Autodesk Inventor part; units mm, degrees
ref_plane "YZ Plane" through (0, 0, 0) normal (1, 0, 0) x (0, 1, 0)
ref_plane "XZ Plane" through (0, 0, 0) normal (0, 1, 0) x (-1, 0, 0)
ref_plane "XY Plane" through (0, 0, 0) normal (0, 0, 1) x (1, 0, 0)
sketch "Esboço1" plane through (0, 0, 0) normal (0, 1, 0) x (-1, 0, 0)
  line L0 (0, 0) -> (0, -150)
  line L1 (0, -150) -> (100, -150)
  line L2 (100, -150) -> (100, 0)
  line L3 (100, 0) -> (0, 0)
  dimension "d0" = 150
  dimension "d1" = 100
extrude "Extrusão1" add sketch "Esboço1" along normal blind 5
fillet "Arredondamento1" radius 5 1 edges at (0, 2.5, 0)
fillet "Arredondamento2" radius 5 1 edges at (-100, 2.5, 0)
fillet "Arredondamento3" radius 5 2 edges at (-100, 2.5, -150) (0, 2.5, -150)
sketch "Esboço2" plane through (0, 5, 0) normal (0, 1, 0) x (1, 0, 0)
  circle A0 centre (-5, 5) radius 2.5
  circle A1 centre (-95, 5) radius 2.5
  circle A2 centre (-68, 145) radius 2.5
  circle A3 centre (-32, 145) radius 2.5
  circle A4 centre (-5, 5) radius 2.5
  dimension "d26" = 5
  dimension "d28" = 5
  dimension "d41" = 5
  dimension "d42" = 5
sketch "Esboço3" plane through (0, 5, 0) normal (0, 1, 0) x (1, 0, 0)
  line L0 (-5, 150) -> (-95, 150)
  line L1 (-80, 108) -> (-80, 63)
  line L2 (-100, 145) -> (-100, 5)
  line L3 (-80, 108) -> (-106.6116, 108)
  line L4 (-80, 63) -> (-106.6116, 63)
  circle A0 centre (-32, 145) radius 2.5
  line L5 (-67.9453, 145) -> (-32, 145)
  point P0 (0, 0)
  point P1 (-100, 108)
  point P2 (-100, 63)
  point P3 (-100, 108)
  point P4 (-100, 63)
  dimension "d53" = 45
extrude "Extrusão9" cut sketch "Esboço3" against normal through all contours L1 L4 L2 L3
extrude "Extrusão10" cut sketch "Esboço2" against normal through all
sketch "Esboço4" plane through (0, 5, 0) normal (0, 1, 0) x (1, 0, 0)
  line L0 (-95, 0) -> (-5, 0)
  line L1 (-5, 34.9997) -> (-42.3, 34.9997)
  line L2 (-42.3, 12.0997) -> (-5, 12.0997)
  line L3 (-42.3, 12.0997) -> (-42.3, 9.7997)
  line L4 (-42.3, 9.7997) -> (-5, 9.7997)
  line L5 (-5, 9.7997) -> (-5, 12.0997)
  line L6 (-5, 34.9997) -> (-5, 37.2997)
  line L7 (-5, 37.2997) -> (-42.3, 37.2997)
  line L8 (-42.3, 37.2997) -> (-42.3, 34.9997)
  line L9 (-57.3, 34.9997) -> (-94.6, 34.9997)
  line L10 (-94.6, 12.0997) -> (-57.3, 12.0997)
  line L11 (-94.6, 12.0997) -> (-94.6, 9.7997)
  line L12 (-94.6, 9.7997) -> (-57.3, 9.7997)
  line L13 (-57.3, 9.7997) -> (-57.3, 12.0997)
  line L14 (-57.3, 34.9997) -> (-57.3, 37.2997)
  line L15 (-57.3, 37.2997) -> (-94.6, 37.2997)
  line L16 (-94.6, 37.2997) -> (-94.6, 34.9997)
  point P0 (0, 0)
  dimension "d62" = 37.3
  dimension "d63" = 22.9
  dimension "d64" = 2.3
  dimension "d65" = 2.3
  dimension "d67" = 37.3
extrude "Extrusão11" cut sketch "Esboço4" against normal through all
properties part number "BaseS"
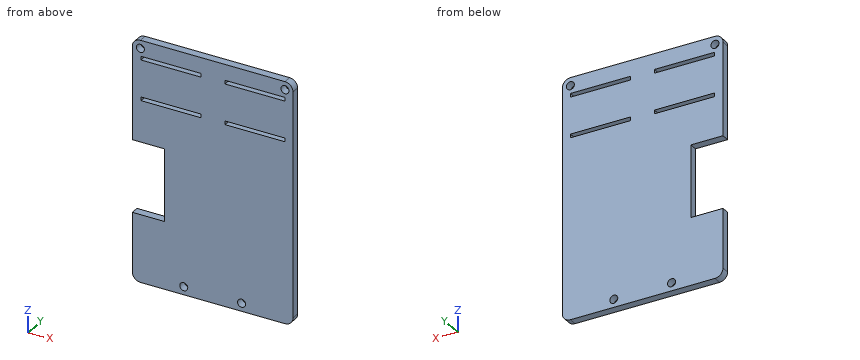
Design review of the part built by this model. Coordinates are the model's own, in mm. Give positions to 0.01 mm unless a question says otherwise; leave off trailing zeros. Loops run counter-clockwise (first coordinate to the right, second up) from the corner with the lowest first, then second, coordinate; pieces in that order, holes last. Notation, with made-up numbers: (56, 66) - (108, 66) arc R30 cw to (108, 91) - close; hole circle Ø8 at (72.5, 87.25). An arc over 180 degrees is marked (long way). Write item = value, one per line.
1) Take a section at D-D on x = -32. State the section outline as (y, z) points, and give its area (3 significant figures).
Result sheet:
outline = (0, -150) - (5, -150) - (5, -147.5) - (0, -147.5) - close; (0, -142.5) - (5, -142.5) - (5, -37.3) - (0, -37.3) - close; (0, -35) - (5, -35) - (5, -12.1) - (0, -12.1) - close; (0, -9.8) - (5, -9.8) - (5, 0) - (0, 0) - close
area = 702 mm2
2) Take a section at A-A on x = -86.5. State the section outline as (y, z) points, and give its area (3 significant figures).
Result sheet:
outline = (0, -150) - (5, -150) - (5, -108) - (0, -108) - close; (0, -63) - (5, -63) - (5, -37.3) - (0, -37.3) - close; (0, -35) - (5, -35) - (5, -12.1) - (0, -12.1) - close; (0, -9.8) - (5, -9.8) - (5, 0) - (0, 0) - close
area = 502 mm2
3) Clearance check with a flat-ended pin moving along its axis: pin 1 Ø4.5 at (x, z) = (-32, -145) entering from -Y. State where the tip first meets the part, or that it passes through.
Result sheet:
pin_1 = through
4) Take a section at C-C on x = -72.5. State the section outline as (y, z) points, and give its area (3 significant figures).
Result sheet:
outline = (0, -150) - (5, -150) - (5, -37.3) - (0, -37.3) - close; (0, -35) - (5, -35) - (5, -12.1) - (0, -12.1) - close; (0, -9.8) - (5, -9.8) - (5, 0) - (0, 0) - close
area = 727 mm2
5) Take a section at B-B on y = 2. Count the separate pieces of the cut face and the enclosed holes in it, and give its area (3 significant figures).
Result sheet:
separate_pieces = 1
enclosed_holes = 8
area = 13,700 mm2
6) To check wall thickness, follow line 1 (X direction, y = 1.1, z = -5); line 2 (X direction, y = 3.75, z = -145); line 3 (Z direction, x = -32, y = 3.5). State the ranges of each line that lie inside material, in increasing order.
Result sheet:
line_1 = -100 to -97.5, -92.5 to -7.5, -2.5 to 0
line_2 = -100 to -70.5, -65.5 to -34.5, -29.5 to 0
line_3 = -150 to -147.5, -142.5 to -37.3, -35 to -12.1, -9.8 to 0
